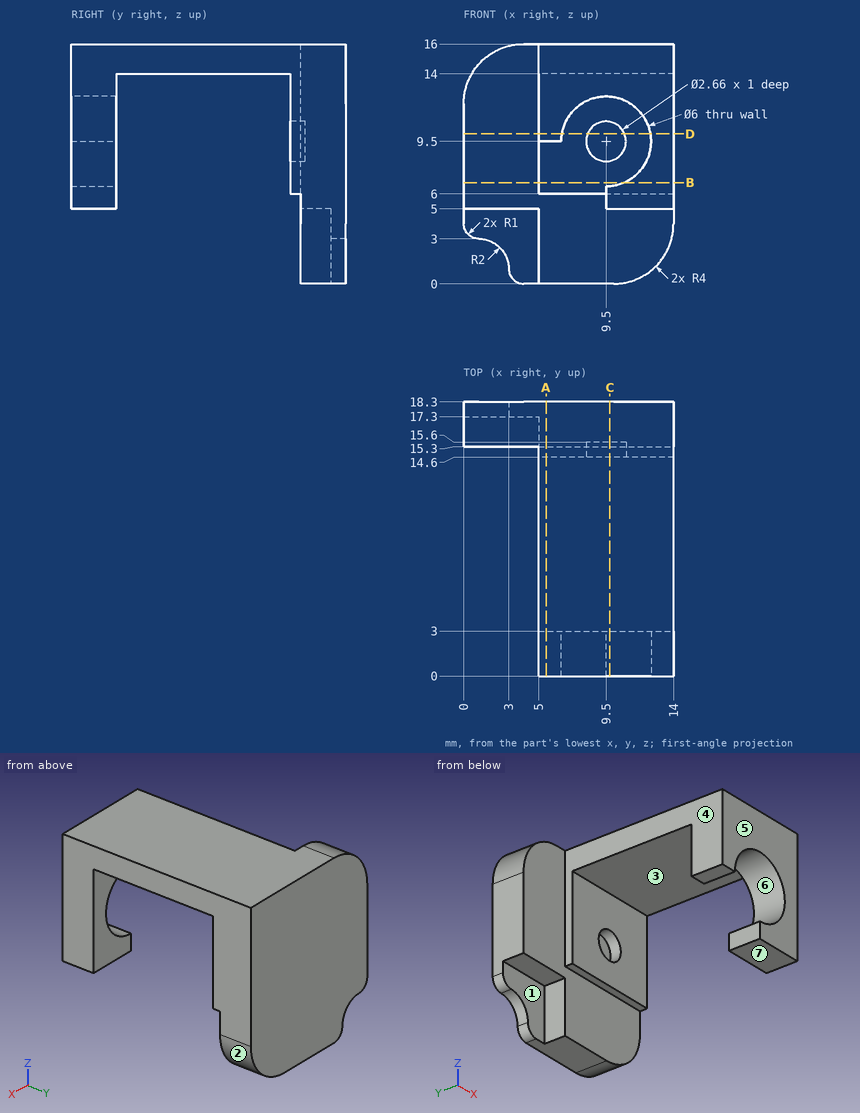
The figure shows three views and two pictorial views of one solid part (mm, origin at its lowest corner). Answer the questions. A direction names the side the tool comes from. Round coordinates to 2 decimals unless told otherwise and drop trailing zeros. Write each loop counter-clockwise with the first axis right and the second up, starting at its lowest first coordinate (ties: lowest second). Pieces come first, ordered by that corner, then holes. Notation, with made-up numbers: (6, 4) - (30, 4) arc R15 cw to (30, 28) - close; hole circle Ø11 at (61, 14.5). An arc over 180 degrees is marked (long way). Answer in a Markdown table with one row per item. Add a question column.
1. Find the intervals of material crossed by line 1 along X through (y, z) = (15, 9.5); line 2 along Y through (x, z) = (7, 13.5); line 3 along Y through (x, z) = (4.5, 11), in increasing order. Write a range as from..to.
2. A cutting plane is placed at A-A, the plane x = 5.5. Determine the outline of the cut face in (y, z).
3. Given pin 1 (2 mm diameter, centred on x = 9.5, z = 9, fed in from -Y); pin 2 (0.6 mm diameter, centred on x = 3, y = 16.5, fed in from -Z); pin 3 (2.5 mm diameter, centred on x = 9.5, z = 9.5, fed in from -Y), each flat-ended and moving along its own axis, determine where each tip first touches the part or whether it passes through.
4. A cutting plane is placed at D-D, the plane z = 10. Determine the outline of the cut face in (x, y).
5. A cutting plane is placed at C-C, the plane x = 9.75. Determine the outline of the cut face in (y, z).
6. For the marked faces 1, 2, 3 and 4, determine the directions among +Z, -Z, +X, -X, +Y, -Y from which every point of the face is accessible in a straight line to the end or side of a thin tool.
7. A cutting plane is placed at B-B, the plane z = 6.75. Determine the outline of the cut face in (x, y).
8. The mould has two halves that part along Z. Classify the marked faces 5, 6 and 7: +Z half, -Z half, draft (parallel to the pull), parting line (faces both ways), or undercut.
Worked out:
| question | item | result |
|---|---|---|
| 1 | line 1 | 5..8.17, 10.83..14 |
| 1 | line 2 | 0..3, 14.6..18.3 |
| 1 | line 3 | 15.3..18.3 |
| 2 | outline | (0, 9.5) - (3, 9.5) - (3, 14) - (14.6, 14) - (14.6, 6) - (15.3, 6) - (15.3, 0) - (18.3, 0) - (18.3, 16) - (0, 16) - close |
| 3 | pin 1 | y = 14.6 |
| 3 | pin 2 | z = 5 |
| 3 | pin 3 | y = 15.6 |
| 4 | outline | (0, 15.3) - (5, 15.3) - (5, 14.6) - (8.27, 14.6) - (8.27, 15.6) - (10.73, 15.6) - (10.73, 14.6) - (14, 14.6) - (14, 18.3) - (0, 18.3) - close; (5, 0) - (6.54, 0) - (6.54, 3) - (5, 3) - close; (12.46, 0) - (14, 0) - (14, 3) - (12.46, 3) - close |
| 5 | outline | (0, 5) - (3, 5) - (3, 6.51) - (0, 6.51) - close; (0, 12.49) - (3, 12.49) - (3, 14) - (14.6, 14) - (14.6, 10.81) - (15.6, 10.81) - (15.6, 8.19) - (14.6, 8.19) - (14.6, 6) - (15.3, 6) - (15.3, 0) - (18.3, 0) - (18.3, 16) - (0, 16) - close |
| 6 | face 1 | -Z, -X, -Y |
| 6 | face 2 | -Z, +X, +Y, -Y |
| 6 | face 3 | -Z, +X, -X |
| 6 | face 4 | +Z, -Z, -X, -Y |
| 7 | outline | (0, 15.3) - (5, 15.3) - (5, 14.6) - (14, 14.6) - (14, 18.3) - (0, 18.3) - close; (10.7, 0) - (14, 0) - (14, 3) - (10.7, 3) - close |
| 8 | face 5 | draft |
| 8 | face 6 | undercut |
| 8 | face 7 | -Z half |
